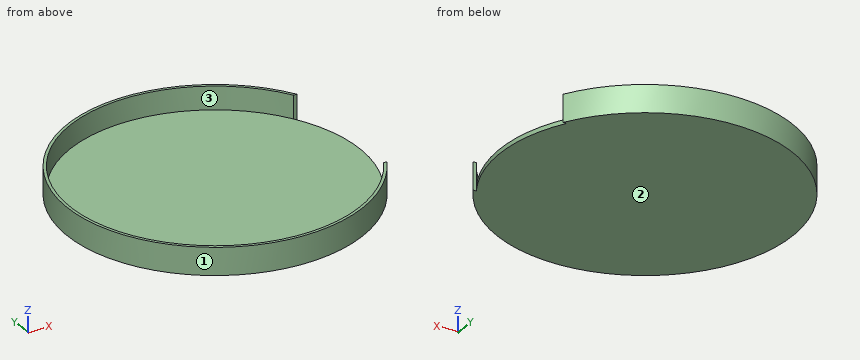
```python
from build123d import *

# Parameters (mm, degrees)
F0_R          = 50
F1_DEPTH      = 1.5
F3_DEPTH      = 8
F3_DEPTH_BACK = 1.5


with BuildPart() as f1:
    # F0 (on Top) → F1 (new body)
    with BuildSketch(Plane.XY):
        with Locations((1.66043, 0)):
            Circle(F0_R)
    extrude(amount=F1_DEPTH)

    # F2 (on face) → F3 (join, two sides)
    with BuildSketch(Plane.XY.offset(1.5)) as f3_sk:
        with BuildLine():
            ThreePointArc((44.9617, -25), (-48.33957, 0), (44.9617, 25))
            Line((44.9617, 25), (46.112651, 25))
            ThreePointArc((46.112651, 25), (-49.33957, 0), (46.112651, -25))
            Line((46.112651, -25), (44.9617, -25))
        make_face()
    extrude(amount=F3_DEPTH)
    extrude(f3_sk.sketch, amount=-F3_DEPTH_BACK)


solid = f1.part
```
Geometry: final body of the model. Coordinates: model frame, mm. Face numbers are marked on the shaded views. Give positions to 0.01 mm unless a question says otherwise; leave off trailing zeros. Loops run counter-clockwise (first coordinate to the right, second up) from the corner with the lowest first, then second, coordinate; pieces in that order, holes last. Notation, with made-up numbers: (-17.75, -12.5) - (-0.75, -12.5) arc R26 cw to (-0.75, 10.5) - close; hole circle Ø6 at (39.5, 57.5). An arc over 180 degrees is marked (long way). Answer as CSV lines item,"result". Start each with the question number.
(1) Ray query, line 1 along X through (y, z) = (0, 3.5); line 2 along Z through (x, y) = (-12, -41); line 3 along X through (y, z) = (36, 3.75). Return the intervals inside material, ascending. Write a range as [from, to].
(2) Section query A-A (y = 0). Output: boundary loops of the cut face in (x, z), and give its area (4 significant figures).
(3) Section query C-C (z = 6.75). Output: boundary loops of the cut face in (x, y), and give its area (3 significant figures).
(4) Section query B-B (x = -25). Output: boundary loops of the cut face in (y, z), and give its area (3 significant figures).
(5) Pin query (flat end, axial travel): P1, Ø2, axis at x = 33.5, y = -19, coming from the -Z side; P2, Ø5, axis at x = -20, y = -17.5, coming from the +Z side; P3, Ø5, axis at x = 22, z = 8, coming from the -Y side; P4, Ø0.6, axis at x = 45.5, z = 3, coming from the -Y side. Return the tip coordinate at first contact, or that it passes through.
(6) Section query D-D (y = -41). Output: boundary loops of the cut face in (x, z).
(7) Mould query, pull axis Y, two halves, no side actions, for the marked faces 1, 2 and 3. Classes: +Y half, -Y half, draft (parallel to the pull), parting line (faces both ways), or undercut.
Worked answers:
1,line 1,"x = [-49.34, -48.34]"
1,line 2,"z = [0, 1.5]"
1,line 3,"x = [-34.46, -33.04], [36.36, 37.79]"
2,outline,"(-49.34, 0) - (51.66, 0) - (51.66, 1.5) - (-48.34, 1.5) - (-48.34, 9.5) - (-49.34, 9.5) - close"
2,area,"159.5 mm^2"
3,outline,"(44.96, -25) arc R50 cw (long way) to (44.96, 25) - (46.11, 25) arc R51 ccw (long way) to (46.11, -25) - close"
3,area,"265 mm^2"
4,outline,"(-43.48, 0) - (43.48, 0) - (43.48, 9.5) - (42.3, 9.5) - (42.3, 1.5) - (-42.3, 1.5) - (-42.3, 9.5) - (-43.48, 9.5) - close"
4,area,"149 mm^2"
5,P1,"stops at z = 0"
5,P2,"stops at z = 1.5"
5,P3,"stops at y = -47.78"
5,P4,"stops at y = -26.56"
6,outline,"(-28.67, 0) - (31.99, 0) - (31.99, 9.5) - (30.28, 9.5) - (30.28, 1.5) - (-26.96, 1.5) - (-26.96, 9.5) - (-28.67, 9.5) - close"
7,face 1,"parting line"
7,face 2,"draft"
7,face 3,"undercut"
